Drawing for the job (mm, zero at the part's lowest x, y, z). Round coordinates to 2 decimals unless told otherwise and drop trailing zeros. Write each loop counter-clockwise with the first axis right and the second up, starting at its lowest first coordinate (ties: lowest second). Pieces come first, ordered by that corner, then holes. Notation, with made-up numbers: (-37.75, -18.5) -> (21.25, -18.5) arc R16 ccw to (21.25, 10.5) -> close; hole circle Ø3 at (81, 81). An arc over 180 degrees is marked (long way). One line per question, with ' | ' between items.
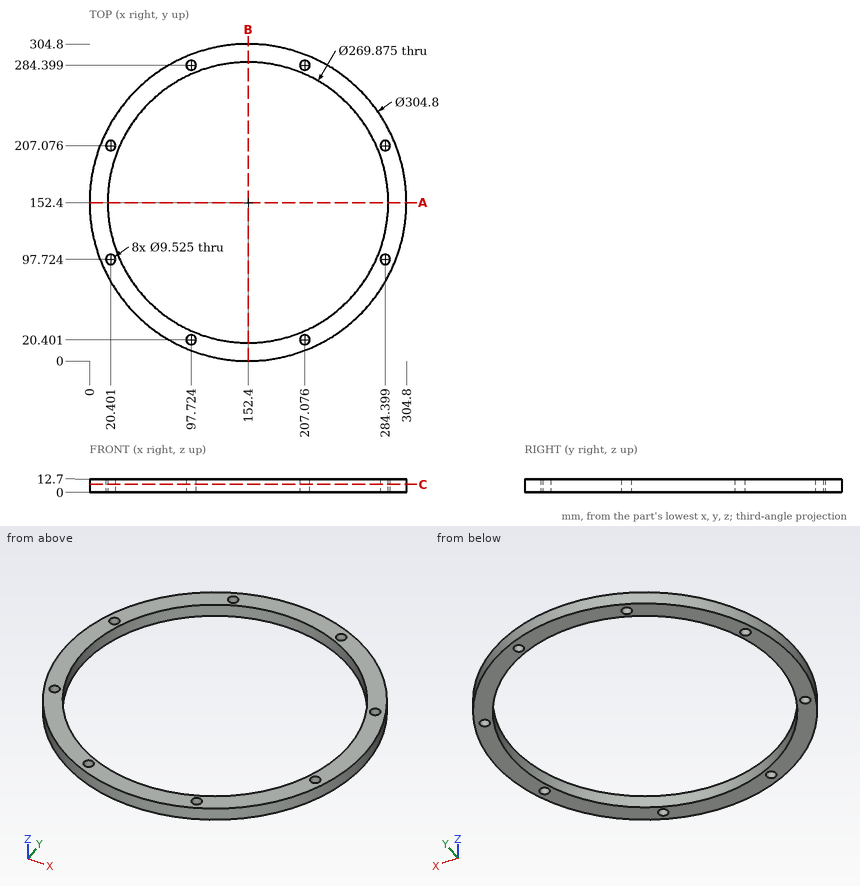
(1) Slice it at C-C (z = 7.5). State how many separate pieces and enclosed holes the cut face has, then the cut area to 3 significant figures.
Calculated:
separate pieces: 1 | enclosed holes: 9 | area: 15,200 mm2
(2) Drop flat-ended pins along their axis: pin 1 (5.5 mm diameter, centred on x = 284.4, y = 207.08, fed in from +Z); pin 2 (6 mm diameter, centred on x = 220, z = 5, fed in from -Y); pin 3 (6 mm diameter, centred on x = 247, y = 38, fed in from -Z); pin 4 (1.5 mm diameter, centred on y = 116.5, z = 6.5, fed in from +X). Give the stop position or say it passes through.
Calculated:
pin 1: through | pin 2: y = 14.37 | pin 3: z = 0 | pin 4: x = 300.69
(3) Slice it at A-A (y = 152.4). Write the cut outline in (x, z).
Calculated:
outline: (0, 0) -> (17.46, 0) -> (17.46, 12.7) -> (0, 12.7) -> close; (287.34, 0) -> (304.8, 0) -> (304.8, 12.7) -> (287.34, 12.7) -> close
(4) Wall check: line 1 (Y direction, x = 85, z = 3.5) (1 decimal); line 2 (X direction, y = 60, z = 9.75) (1 decimal); line 3 (Y direction, x = 242, z = 11) (1 decimal). Give the ranges that are in metal, low to high. Write a range as from..to.
Calculated:
line 1: 15.7..35.5, 269.3..289.1 | line 2: 31.2..54.1, 250.7..273.6 | line 3: 29.1..51.5, 253.3..275.7
